```python
from build123d import *

# Parameters (mm, degrees)
BOSS_EXTRUDE1_DEPTH = 285.75
SKETCH2_W           = 177.8
SKETCH2_H           = 76.2
CUT_EXTRUDE1_DEPTH  = 40.7002
CUT_EXTRUDE2_REACH  = 41.7
SKETCH3_R           = 2.2479


with BuildPart() as part:
    # Sketch1 → Boss-Extrude1 (new body)
    with BuildSketch(Plane.XY):
        Polygon((0, 0), (0, 279.4), (63.5, 389.385226281), (64.885813851, 388.585126281), (1.6002, 278.971227702), (1.6002, 0), (1.6002, -1.6002), (0, -1.6002), (-38.1, -1.6002), (-38.1, 0), align=None)
    extrude(amount=BOSS_EXTRUDE1_DEPTH)

    # Sketch2 → Cut-Extrude1 (cut, through all)
    with BuildSketch(Plane(origin=(1.6002, 0, 0), x_dir=(0, 0, -1), z_dir=(1, 0, 0))):
        with Locations((-142.875, 95.25)):
            Rectangle(SKETCH2_W, SKETCH2_H)
    extrude(amount=-CUT_EXTRUDE1_DEPTH, mode=Mode.SUBTRACT)

    # Sketch3 → Cut-Extrude2 (cut, up to next)
    with BuildSketch(Plane(origin=(1.6002, 0, 0), x_dir=(0, 0, -1), z_dir=(1, 0, 0)), mode=Mode.PRIVATE) as cut_extrude2_sk1:
        with Locations((-268.762499939, 215.471227702)):
            Circle(SKETCH3_R)
    cut_extrude2_tool1 = extrude(cut_extrude2_sk1.sketch, amount=-CUT_EXTRUDE2_REACH, mode=Mode.PRIVATE) & part.part
    add(cut_extrude2_tool1.solids().sort_by_distance((1.6002, 215.471228, 268.7625))[0], mode=Mode.SUBTRACT)
    # Sketch3 → Cut-Extrude2 (cut, up to next)
    with BuildSketch(Plane(origin=(1.6002, 0, 0), x_dir=(0, 0, -1), z_dir=(1, 0, 0)), mode=Mode.PRIVATE) as cut_extrude2_sk2:
        with Locations((-248.762500061, 215.471227702)):
            Circle(SKETCH3_R)
    cut_extrude2_tool2 = extrude(cut_extrude2_sk2.sketch, amount=-CUT_EXTRUDE2_REACH, mode=Mode.PRIVATE) & part.part
    add(cut_extrude2_tool2.solids().sort_by_distance((1.6002, 215.471228, 248.7625))[0], mode=Mode.SUBTRACT)
    # Sketch3 → Cut-Extrude2 (cut, up to next)
    with BuildSketch(Plane(origin=(1.6002, 0, 0), x_dir=(0, 0, -1), z_dir=(1, 0, 0)), mode=Mode.PRIVATE) as cut_extrude2_sk3:
        with Locations((-16.987500061, 215.471227702)):
            Circle(SKETCH3_R)
    cut_extrude2_tool3 = extrude(cut_extrude2_sk3.sketch, amount=-CUT_EXTRUDE2_REACH, mode=Mode.PRIVATE) & part.part
    add(cut_extrude2_tool3.solids().sort_by_distance((1.6002, 215.471228, 16.9875))[0], mode=Mode.SUBTRACT)
    # Sketch3 → Cut-Extrude2 (cut, up to next)
    with BuildSketch(Plane(origin=(1.6002, 0, 0), x_dir=(0, 0, -1), z_dir=(1, 0, 0)), mode=Mode.PRIVATE) as cut_extrude2_sk4:
        with Locations((-36.987499939, 215.471227702)):
            Circle(SKETCH3_R)
    cut_extrude2_tool4 = extrude(cut_extrude2_sk4.sketch, amount=-CUT_EXTRUDE2_REACH, mode=Mode.PRIVATE) & part.part
    add(cut_extrude2_tool4.solids().sort_by_distance((1.6002, 215.471228, 36.9875))[0], mode=Mode.SUBTRACT)


solid = part.part
```
Could you check a few things on this model? Use its own coordinates, in mm. A direction names the side the tool comes from. Round coordinates to 2 decimals unless told otherwise and drop trailing zeros. Loops run counter-clockwise (first coordinate to the right, second up) from the corner with the lowest first, then second, coordinate; pieces in that order, holes last.
Q1. I want a section at A-A (y = 106). Write out the boundary of the cut face in (x, z) (3 decimals).
Q2. On a 3-axis mill with a long thin cutter (end or side, diameter ignored), from which of +Z, -Z, +X, -X, +Y, -Y can I reach the whole of each face in a straight line? I mean faces 1 (the flat face through (1.6, 137, 141)), 2 (the flat face through (0, 138, 141)), 3 (the flat face through (-19, -1.6, 141)). Say none if no direction works.
Q3. I want a section at C-C (y = 187). Write out the boundary of the cut face in (x, z).
Q4. I want a section at B-B (z = 175). Write out the boundary of the cut face in (x, y).
Q5. For P1, Ø3, axis at x = 43, z = 136.5, coming from the -Y side; P2, Ø19, axis at x = -26.5, z = 71.5, coming from the +Y side; P3, Ø3, axis at x = 25, z = 163, coming from the -Y side; P4, Ø4, axis at y = 215.47, z = 36.99, coming from the +X side, each with a flat end and sliding along its axis, tell me the tip position at first contact or that it passes through.
Q6. I want a section at D-D (x = -19). Write out the boundary of the cut face in (y, z).
Q7. Please list where these lines run through material, in increasing order: L1, parallel to X at y = 271, z = 103.5; L2, parallel to Y at x = -22, z = 224.5; L3, parallel to X at y = 322, z = 241.5.
Answer below:
1. outline: (0, 0) - (1.6, 0) - (1.6, 53.975) - (0, 53.975) - close; (0, 231.775) - (1.6, 231.775) - (1.6, 285.75) - (0, 285.75) - close
2. face 1: +Z, -Z, +X, -Y
2. face 2: +Z, -Z, -X, +Y
2. face 3: +Z, -Z, +X, -X, -Y
3. outline: (0, 0) - (1.6, 0) - (1.6, 285.75) - (0, 285.75) - close
4. outline: (-38.1, -1.6) - (1.6, -1.6) - (1.6, 57.15) - (0, 57.15) - (0, 0) - (-38.1, 0) - close; (0, 133.35) - (1.6, 133.35) - (1.6, 278.97) - (64.89, 388.59) - (63.5, 389.39) - (0, 279.4) - close
5. P1: stops at y = 348.08
5. P2: stops at y = 0
5. P3: stops at y = 316.9
5. P4: passes through
6. outline: (-1.6, 0) - (0, 0) - (0, 285.75) - (-1.6, 285.75) - close
7. L1: x = 0 to 1.6
7. L2: y = -1.6 to 0
7. L3: x = 24.6 to 26.44
